Work out the finished part from the listing and answer in its coordinate system (mm). A direction names the side the tool comes from. Coordinates: 2 decimals unless noted, no trailing zeros. Write each loop counter-clockwise with the first axis right and the second up, starting at its lowest first coordinate (ties: lowest second). Pieces come first, ordered by that corner, then holes. Notation, with made-up numbers: M 24,77.5 L 71,77.5 A16 ccw 71,105.5 Z; hole C 22.25,77.5 d2. An arc over 180 degrees is marked long. Use CSV: the item, a comma, the result in double quotes.
Autodesk Inventor part; units mm, degrees
ref_plane "YZ Plane" through (0, 0, 0) normal (1, 0, 0) x (0, 1, 0)
ref_plane "XZ Plane" through (0, 0, 0) normal (0, 1, 0) x (-1, 0, 0)
ref_plane "XY Plane" through (0, 0, 0) normal (0, 0, 1) x (1, 0, 0)
sketch "Sketch1" plane through (0, 0, 0) normal (0, 0, 1) x (1, 0, 0)
  line L0 (-12.7, 0) -> (12.7, 0) construction
  line L1 (12.7, 0) -> (12.7, -57.15)
  line L2 (12.7, -57.15) -> (-12.7, -57.15)
  line L3 (-12.7, -57.15) -> (-12.7, 0) construction
  line L4 (-35.1269, 0) -> (-12.7, -11.9246) construction
  line L5 (-12.7, -11.9246) -> (-36.5492, -56.7783)
  line L6 (-36.5492, -56.7783) -> (-58.976, -44.8537)
  line L7 (-58.976, -44.8537) -> (-35.1269, 0)
  line L8 (-23.9134, -5.9623) -> (-47.7626, -50.816) construction
  line L9 (-35.1269, 0) -> (12.7, 0)
  line L10 (-12.7, -11.9246) -> (-12.7, -57.15)
  point P0 (0, 0)
  point P1 (0, 0)
  point P2 (-29.8757, -17.1757)
  point P3 (-41.8003, -39.6026)
  point P4 (0, -12.7)
  point P5 (0, -38.1)
  dimension "d0" = 25.4
  dimension "d1" = 25.4
  dimension "d2" = 28
  dimension "d3" = 50.8
  dimension "d4" = 25.4
  dimension "d5" = 12.7
  dimension "d6" = 25.4
  dimension "d7" = 12.7
  dimension "d8" = 57.15
extrude "Extrusion1" add sketch "Sketch1" against normal blind 6.35
hole "Hole1" at (-29.8757, -17.1757, 0) at (-41.8003, -39.6026, 0) at (0, -12.7, 0) at (0, -38.1, 0) direction (0, 0, -1) diameter 5.1054 end through all
fillet "Fillet1" radius 6.35 7 edges at (12.7, 0, -3.175) (12.7, -57.15, -3.175) (-12.7, -57.15, -3.175) (-12.7, -11.9246, -3.175) (-36.5492, -56.7783, -3.175) (-58.976, -44.8537, -3.175) (-35.1269, 0, -3.175)
properties part number "CL4-009" material "Aluminum 6061"
Item 1: Given pin 1 (1.5 mm diameter, centred on x = -33.5, z = -3, fed in from +Y); pin 2 (4.5 mm diameter, centred on x = -41.8, y = -39.6, fed in from +Z); pin 3 (1.9 mm diameter, centred on y = -44.5, z = -4.5, fed in from -X); pin 4 (1.5 mm diameter, centred on x = -10.5, z = -1, fed in from -Y), each flat-ended and moving along its own axis, determine where each tip first touches the part or whether it passes through.
Answer:
pin 1,"stops at y = -0.17"
pin 2,"passes through"
pin 3,"stops at x = -56.6"
pin 4,"stops at y = -56.16"
Item 2: The part is cut by section D-D (y = -25.5). Write down the section's boundary in (x, z).
Answer:
outline,"M -48.69,-6.35 L 12.7,-6.35 L 12.7,0 L -48.69,0 Z"
Item 3: A tool of negligible diameter and unlimited length cuts with its end or side. For faces 1 (the face through (12.7, -28, -3)), 2 (the face through (-10.79, -55.34, -3.22)), from which of +Z, -Z, +X, -X, +Y, -Y can it reach the whole face along a straight path? Write none if from no direction.
Answer:
face 1,"+Z, -Z, +X, +Y, -Y"
face 2,"+Z, -Z, -Y"
Item 4: Consider probe 1 along Y at (x, z) = (0, -1.5); probe 2 along X at (y, z) = (-38.1, -1.25) (3 decimals); probe 3 along Y at (x, z) = (2, -4.5). Determine where each line is inside the solid, lowest interval first.
Answer:
probe 1,"y = -57.15 to -40.65, -35.55 to -15.25, -10.15 to 0"
probe 2,"x = -55.385 to -43.864, -39.737 to -26.618, -12.7 to -2.553, 2.553 to 12.7"
probe 3,"y = -57.15 to -39.69, -36.51 to -14.29, -11.11 to 0"
Item 5: For a pull along X with two mould halves and no side action, classify faces 3 (the face through (10.89, -55.24, -3.22)), 4 (the face through (-46.59, -21.56, -3.13)), 5 (the face through (-0.767, -40.535, -3.219)) as released by +X, released by -X, zero draft, split by the parting line, or undercut.
Answer:
face 3,"released by +X"
face 4,"released by -X"
face 5,"undercut"
Item 6: The part is cut by section A-A (x = 0). Write down the section's boundary in (y, z).
Answer:
outline,"M -57.15,-6.35 L -40.65,-6.35 L -40.65,0 L -57.15,0 Z; M -35.55,-6.35 L -15.25,-6.35 L -15.25,0 L -35.55,0 Z; M -10.15,-6.35 L 0,-6.35 L 0,0 L -10.15,0 Z"
Item 7: The part is cut by section C-C (z = -4.75). Write down the section's boundary in (x, y), then the cut area to 3 significant figures.
Answer:
outline,"M -55.99,-39.25 A6.35 ccw -53.37,-47.83 L -42.16,-53.8 A6.35 ccw -33.57,-51.17 L -24.66,-34.41 A6.35 cw -12.7,-37.39 L -12.7,-50.8 A6.35 ccw -6.35,-57.15 L 6.35,-57.15 A6.35 ccw 12.7,-50.8 L 12.7,-6.35 A6.35 ccw 6.35,0 L -31.31,0 A6.35 ccw -36.92,-3.37 Z; hole C -41.8,-39.6 d5.11; hole C -29.88,-17.18 d5.11; hole C 0,-38.1 d5.11; hole C 0,-12.7 d5.11"
area,"2,860 mm2"
Item 8: The part is cut by section B-B (y = -13.5). Write down the section's boundary in (x, z), then the cut area to 3 significant figures.
Answer:
outline,"M -42.3,-6.35 L -2.42,-6.35 L -2.42,0 L -42.3,0 Z; M 2.42,-6.35 L 12.7,-6.35 L 12.7,0 L 2.42,0 Z"
area,"318 mm2"
